Autodesk Inventor part; units mm, degrees
ref_plane "Work Plane1" through (-165, 8, 47) normal (0, 0, 1) x (1, 0, 0)
ref_plane "Work Plane2" through (29.9285, 8, 9) normal (-1, 0, 0) x (0, 0, 1)
ref_plane "Work Plane3" through (64.9709, 8, 15.5) normal (-1, 0, 0) x (0, 0, 1)
sketch "Sketch1" plane through (0, 0, 0) normal (0, 1, 0) x (-1, 0, 0)
  line L0 (-165, 47) -> (-165, 8)
  line L1 (165, 8) -> (165, 47)
  line L2 (-78, 0) -> (95.3, 0)
  line L3 (95.3, 0) -> (95.3, 15)
  line L4 (95.3, 15) -> (115.5, 15)
  line L5 (115.5, 15) -> (115.5, 0)
  line L6 (-115.5, 0) -> (-115.5, 15)
  line L7 (-115.5, 15) -> (-95.3, 15)
  line L8 (-95.3, 15) -> (-95.3, 0)
  line L9 (125, 47) -> (122, 44)
  line L10 (122, 44) -> (-122, 44)
  line L11 (-122, 44) -> (-125, 47)
  line L12 (0, 0) -> (0, 44) construction
  line L13 (165, 47) -> (125, 47)
  line L14 (-125, 47) -> (-165, 47)
  line L15 (115.5, 0) -> (157, 0)
  line L16 (-157, 0) -> (-115.5, 0)
  line L17 (-95.3, 0) -> (95.3, 0)
  line L18 (155.4, 11) -> (146.9, 11)
  line L19 (146.9, 11) -> (146.9, 32)
  line L20 (146.9, 32) -> (155.4, 32)
  line L21 (155.4, 32) -> (155.4, 11)
  line L22 (-146.9, 11) -> (-155.4, 11)
  line L23 (-155.4, 11) -> (-155.4, 32)
  line L24 (-155.4, 32) -> (-146.9, 32)
  line L25 (-146.9, 32) -> (-146.9, 11)
  line L26 (77, 15) -> (68.5, 15)
  line L27 (68.5, 15) -> (68.5, 23.5)
  line L28 (68.5, 23.5) -> (77, 23.5)
  line L29 (77, 23.5) -> (77, 15)
  line L30 (-25.6785, 15.5) -> (-34.1785, 15.5)
  line L31 (-34.1785, 15.5) -> (-34.1785, 27.5)
  line L32 (-34.1785, 27.5) -> (-25.6785, 27.5)
  line L33 (-25.6785, 27.5) -> (-25.6785, 15.5)
  line L34 (-60.7209, 15.5) -> (-69.2209, 15.5)
  line L35 (-69.2209, 15.5) -> (-69.2209, 31.5)
  line L36 (-69.2209, 31.5) -> (-60.7209, 31.5)
  line L37 (-60.7209, 31.5) -> (-60.7209, 15.5)
  arc A0 (157, 0) -> (165, 8) centre (157, 8) ccw
  arc A1 (-165, 8) -> (-157, 0) centre (-157, 8) ccw
  dimension "d0" = 330
  dimension "d1" = 47
  dimension "d2" = 45
  dimension "d3" = 3
  dimension "d4" = 40
  dimension "d5" = 49.5
  dimension "d6" = 20.2
  dimension "d8" = 15
  dimension "d9" = 11
  dimension "d10" = 9.6
  dimension "d11" = 8.5
  dimension "d12" = 21
  dimension "d13" = 8.5
  dimension "d14" = 8.5
  dimension "d15" = 8.5
  dimension "d16" = 12
  dimension "d17" = 8.5
  dimension "d18" = 16
  dimension "d19" = 95.7791
  dimension "d20" = 130.8215
  dimension "d21" = 88
  dimension "d22" = 15
  dimension "d23" = 15.5
  dimension "d24" = 15.5
  dimension "d25" = 8
extrude "Extrusion1" add sketch "Sketch1" along normal blind 8
fillet "Fillet1" radius 2 8 edges at (-115.5, 4, 0) (-95.3, 4, 0) (95.3, 4, 0) (115.5, 4, 0) (-125, 4, 47) (-122, 4, 44) (122, 4, 44) (125, 4, 47)
sketch "Sketch2" plane through (0, 8, 0) normal (0, 1, 0) x (1, 0, 0)
  arc A0 (124.4142, -46.4142) -> (125.8284, -47) centre (125.8284, -45) ccw construction
  line L0 (125.8284, -47) -> (165, -47) construction
  line L1 (165, -47) -> (165, -8) construction
  arc A1 (165, -8) -> (157, 0) centre (157, -8) ccw construction
  line L2 (157, 0) -> (117.5, 0) construction
  arc A2 (117.5, 0) -> (115.5, -2) centre (117.5, -2) ccw construction
  line L3 (115.5, -2) -> (115.5, -15) construction
  line L4 (115.5, -15) -> (95.3, -15) construction
  line L5 (95.3, -15) -> (95.3, -2) construction
  arc A3 (95.3, -2) -> (93.3, 0) centre (93.3, -2) ccw construction
  line L6 (93.3, 0) -> (-93.3, 0) construction
  arc A4 (-93.3, 0) -> (-95.3, -2) centre (-93.3, -2) ccw construction
  line L7 (-95.3, -2) -> (-95.3, -15) construction
  line L8 (-95.3, -15) -> (-115.5, -15) construction
  line L9 (-115.5, -15) -> (-115.5, -2) construction
  arc A5 (-115.5, -2) -> (-117.5, 0) centre (-117.5, -2) ccw construction
  line L10 (-117.5, 0) -> (-157, 0) construction
  arc A6 (-157, 0) -> (-165, -8) centre (-157, -8) ccw construction
  line L11 (-165, -8) -> (-165, -47) construction
  line L12 (-165, -47) -> (-125.8284, -47) construction
  arc A7 (-125.8284, -47) -> (-124.4142, -46.4142) centre (-125.8284, -45) ccw construction
  line L13 (-124.4142, -46.4142) -> (-122.5858, -44.5858) construction
  arc A8 (-121.1716, -44) -> (-122.5858, -44.5858) centre (-121.1716, -46) ccw construction
  line L14 (-121.1716, -44) -> (121.1716, -44) construction
  arc A9 (122.5858, -44.5858) -> (121.1716, -44) centre (121.1716, -46) ccw construction
  line L15 (122.5858, -44.5858) -> (124.4142, -46.4142) construction
  line L16 (155.4, -11) -> (155.4, -32) construction
  line L17 (155.4, -32) -> (146.9, -32) construction
  line L18 (146.9, -32) -> (146.9, -11) construction
  line L19 (146.9, -11) -> (155.4, -11) construction
  line L20 (-146.9, -11) -> (-146.9, -32) construction
  line L21 (-146.9, -32) -> (-155.4, -32) construction
  line L22 (-155.4, -32) -> (-155.4, -11) construction
  line L23 (-155.4, -11) -> (-146.9, -11) construction
  line L24 (69.2209, -15.5) -> (69.2209, -31.5) construction
  line L25 (69.2209, -31.5) -> (60.7209, -31.5) construction
  line L26 (60.7209, -31.5) -> (60.7209, -15.5) construction
  line L27 (60.7209, -15.5) -> (69.2209, -15.5) construction
  line L28 (34.1785, -15.5) -> (34.1785, -27.5) construction
  line L29 (34.1785, -27.5) -> (25.6785, -27.5) construction
  line L30 (25.6785, -27.5) -> (25.6785, -15.5) construction
  line L31 (25.6785, -15.5) -> (34.1785, -15.5) construction
  line L32 (-68.5, -15) -> (-68.5, -23.5) construction
  line L33 (-68.5, -23.5) -> (-77, -23.5) construction
  line L34 (-77, -23.5) -> (-77, -15) construction
  line L35 (-77, -15) -> (-68.5, -15) construction
  line L36 (-165, -47) -> (-125.8284, -47) construction
  line L37 (-151.15, -47) -> (-151.15, 0) construction
  line L38 (151.15, 0) -> (151.15, -47) construction
  line L39 (29.9285, -9) -> (29.9285, -37.5) construction
  line L40 (64.9709, -15.5) -> (64.9709, -37.5) construction
  line L41 (-77, -23.5) -> (-77, -15) construction
  line L42 (-77, -19.25) -> (-59, -19.25) construction
  point P0 (0, 0)
  point P1 (-151.15, -11)
  point P2 (151.15, -11)
  point P3 (151.15, -6)
  point P4 (151.15, -37)
  point P5 (-151.15, -6)
  point P6 (-151.15, -37)
  point P7 (71, -6.5)
  point P8 (85.75, -6.5)
  point P9 (109, -24)
  point P10 (132, -38)
  point P11 (132, -25.5)
  point P12 (-85.75, -6.5)
  point P13 (-71, -6.5)
  point P14 (-109, -24)
  point P15 (29.9285, -27.5)
  point P16 (29.9285, -15.5)
  point P17 (-21.5, -25)
  dimension "d29" = 5
  dimension "d30" = 5
  dimension "d31" = 5
  dimension "d32" = 5
  dimension "d33" = 6.5
  dimension "d34" = 10
  dimension "d35" = 6
  dimension "d36" = 6.5
  dimension "d37" = 33
  dimension "d38" = 9
  dimension "d39" = 21.5
  dimension "d40" = 79.25
  dimension "d41" = 94
  dimension "d42" = 94
  dimension "d43" = 79.25
  dimension "d44" = 9.5
  dimension "d45" = 56
  dimension "d46" = 56
  dimension "d47" = 24
  dimension "d48" = 24
  dimension "d56" = 143.5
  dimension "d57" = 25
hole "Hole1" at (151.15, 8, 6) at (151.15, 8, 37) at (-151.15, 8, 6) at (-151.15, 8, 37) at (29.9285, 8, 9) at (29.9285, 8, 37.5) at (64.9709, 8, 37.5) at (71, 8, 6.5) at (132, 8, 38) at (-71, 8, 6.5) at (-59, 8, 19.25) direction (0, -1, 0) diameter 3.5 end through all
hole "Hole2" at (85.75, 8, 6.5) at (109, 8, 24) at (-85.75, 8, 6.5) at (-109, 8, 24) direction (0, -1, 0) diameter 8.5 end through all
hole "Hole3" at (-21.5, 8, 25) direction (0, -1, 0) diameter 20.5 end through all
hole "Hole4" at (132, 8, 25.5) direction (0, -1, 0) diameter 16.5 end through all
ref_plane "Work Plane1" through (-165, 8, 47) normal (0, 0, 1) x (1, 0, 0)
ref_plane "Work Plane2" through (29.9285, 8, 9) normal (-1, 0, 0) x (0, 0, 1)
ref_plane "Work Plane3" through (64.9709, 8, 15.5) normal (-1, 0, 0) x (0, 0, 1)
properties part number "A8-0009"
Input: part model. Units: mm. Frame: model coordinates. A direction names the side the tool comes from. Give positions to 0.01 mm unless a question says otherwise; leave off trailing zeros. Loops run counter-clockwise (first coordinate to the right, second up) from the corner with the lowest first, then second, coordinate; pieces in that order, holes last. Notation, with made-up numbers: M -28,7.25 L -4,7.25 A17 ccw -4,21.25 Z; hole C 84.25,11.5 d11. An arc over 180 degrees is marked long. Use one line per item in the form item = value.
1. Reachability of faces 1 (the face through (-73, 4, 23.5)), 2 (the face through (106, 4, 15)), 3 (the face through (1, 4, 0)) from +Z, -Z, +X, -X, +Y, -Y: full face, straight path, thin tool, end or side. Return the list, or none.
Numbers:
face_1 = +Y, -Y
face_2 = -Z, +Y, -Y
face_3 = -Z, +X, -X, +Y, -Y
2. Pull-direction query (X, two-part tool) for faces 4 (the face through (162.594, 3.944, 2.281)), 5 (the face through (-165, 4, 27)), 6 (the face through (34.178, 4, 21)), 7 (the face through (-115.5, 4, 9)); classes: released by +X, released by -X, zero draft, split by the parting line, or undercut.
Numbers:
face_4 = released by +X
face_5 = released by -X
face_6 = undercut
face_7 = undercut
3. First-contact query: pin 1 (3 mm diameter, centred on x = 29.93, z = 9, fed in from -Y); pin 2 (2.5 mm diameter, centred on x = -19, y = 6, fed in from +Z). Flat tips, straight axial feed; report the tip coordinate or a pass-through.
Numbers:
pin_1 = through
pin_2 = 44
4. Line query: L1, parallel to Z at x = -71, y = 5.5; L2, parallel to Z at x = 132, y = 6; L3, parallel to Z at x = -21.5, y = 5. Output: solid intervals per line, ascending.
Numbers:
L1 = 0 to 4.75, 8.25 to 15, 23.5 to 44
L2 = 0 to 17.25, 33.75 to 36.25, 39.75 to 47
L3 = 0 to 14.75, 35.25 to 44
5. Section query A-A, the plane x = 85.75. Return the cut outline in (y, z), and give its area (3 significant figures).
Numbers:
outline = M 0,0 L 8,0 L 8,2.25 L 0,2.25 Z; M 0,10.75 L 8,10.75 L 8,44 L 0,44 Z
area = 284 mm²
6. Section query B-B, the plane y = 1.75. Count the separate pieces of the cut face and the enclosed holes in it, and give its area (3 significant figures).
Numbers:
separate_pieces = 1
enclosed_holes = 22
area = 12,600 mm²
